The listing builds one solid part. Answer for the finished solid, in the listing's coordinates (mm). Face numbers are marked on the shaded views. A direction names the side the tool comes from. Coordinates: 2 decimals unless noted, no trailing zeros. Order: outer loops, then holes, each group sorted by start corner. A loop starts at its lowest first (then second) coordinate and runs counter-clockwise, first axis right, second up. Notation, with made-up numbers: (20.25, 42) -> (28.25, 42) arc R25 cw to (28.25, 63) -> close; hole circle Ø2 at (56, -9.5). An arc over 180 degrees is marked (long way). Return JSON: item names as keys, results as strings.
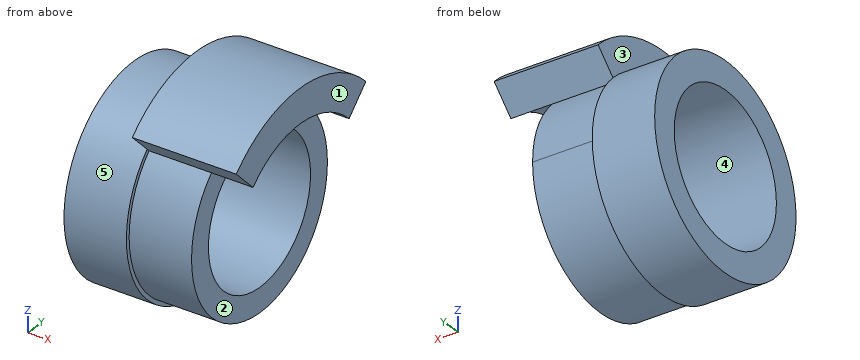
```python
from build123d import *

# Parameters (mm, degrees)
F0_R     = 38.75
F0_R_2   = 28
F1_DEPTH = 48
F5_DEPTH = 40


with BuildPart() as f1:
    # F0 (on Right) → F1 (new body)
    with BuildSketch(Plane.YZ):
        Circle(F0_R)
        Circle(F0_R_2, mode=Mode.SUBTRACT)
    extrude(amount=F1_DEPTH)

    # F2 (on Front) → F3 (revolve)
    with BuildSketch(Plane.XZ):
        Polygon((24, 50.25), (24, 38.75), (48, 38.75), (48, 37.25), (64, 37.25), (64, 50.25), align=None)
    revolve(axis=Axis((48, 0, 0), (1, 0, 0)))

    # F4 (on face) → F5 (cut)
    with BuildSketch(Plane.YZ.offset(64)):
        with BuildLine():
            ThreePointArc((37.25, 0), (-14.2549578556, -34.414512586), (-26.3397275992, 26.3397275992))
            Line((-26.3397275992, 26.3397275992), (-35.5321157546, 35.5321157546))
            ThreePointArc((-35.5321157546, 35.5321157546), (-19.2298424763, -46.4249465087), (50.25, 0))
            ThreePointArc((50.25, 0), (46.4249465087, 19.2298424763), (35.5321157546, 35.5321157546))
            Line((35.5321157546, 35.5321157546), (26.3397275992, 26.3397275992))
            ThreePointArc((26.3397275992, 26.3397275992), (34.414512586, 14.2549578556), (37.25, 0))
        make_face()
    extrude(amount=-F5_DEPTH, mode=Mode.SUBTRACT)


solid = f1.part
```
Item 1: The part is cut by section D-D on y = 22. Determine the outline of the cut face in (x, z), plus the area to 3 significant figures.
Answer list:
{"outline": "(0, -31.9) -> (24, -31.9) -> (24, -30.06) -> (48, -30.06) -> (48, -17.32) -> (0, -17.32) -> close; (0, 17.32) -> (48, 17.32) -> (48, 30.06) -> (64, 30.06) -> (64, 45.18) -> (24, 45.18) -> (24, 31.9) -> (0, 31.9) -> close", "area": "1,920 mm2"}
Item 2: Find the intervals of material crossed by probe 1 along Z at (x, y) = (22, 0); probe 2 along Z at (x, y) = (34.5, 0); probe 3 along X at (y, z) = (-4, -28), in increasing order.
Answer list:
{"probe 1": "-38.75 to -28, 28 to 38.75", "probe 2": "-37.25 to -28, 28 to 50.25", "probe 3": "0 to 48"}
Item 3: Determine the mould class of the marked faces 3, 4 and 5 for opening direction Z: pulls with the +Z half, pulls with the -Z half, needs draft (parallel to the pull), parting line crosses it, or undercut.
Answer list:
{"face 3": "needs draft", "face 4": "undercut", "face 5": "parting line crosses it"}
Item 4: Which of the six approach directions +Z, -Z, +X, -X, +Y, -Y give full straight-line access (tool end or side, diameter ignored) to the marked faces 1 and 2?
Answer list:
{"face 1": "+Z, -Z, +X, +Y, -Y", "face 2": "-Z, +X"}
Item 5: Flat-ended cylindrical pins translate along their axes: pin 1 (12 mm diameter, centred on x = 46.5, y = -15.5, fed in from -Z); pin 2 (22.5 mm diameter, centred on y = 8, z = -15.5, fed in from +X); pin 3 (12 mm diameter, centred on x = 34, z = -22.5, fed in from +Y). Find the tip coordinate at first contact, or state that the pin passes through.
Answer list:
{"pin 1": "z = -36.02", "pin 2": "x = 48", "pin 3": "y = 33.4"}
Item 6: The part is cut by section B-B on z = -5. Determine the outline of the cut face in (x, y), plus the area to 3 significant figures.
Answer list:
{"outline": "(0, -38.43) -> (24, -38.43) -> (24, -36.91) -> (48, -36.91) -> (48, -27.55) -> (0, -27.55) -> close; (0, 27.55) -> (48, 27.55) -> (48, 36.91) -> (24, 36.91) -> (24, 38.43) -> (0, 38.43) -> close", "area": "971 mm2"}
Item 7: The part is cut by section C-C on x = 25.5. Determine the outline of the cut face in (y, z).
Answer list:
{"outline": "(-35.53, 35.53) -> (-26.34, 26.34) arc R37.25 ccw (long way) to (26.34, 26.34) -> (35.53, 35.53) arc R50.25 ccw to start; hole circle Ø56 at (0, 0)"}
Item 8: The part is cut by section A-A on y = 0. Determine the outline of the cut face in (x, z), plus the area to 3 significant figures.
Answer list:
{"outline": "(0, -38.75) -> (24, -38.75) -> (24, -37.25) -> (48, -37.25) -> (48, -28) -> (0, -28) -> close; (0, 28) -> (48, 28) -> (48, 37.25) -> (64, 37.25) -> (64, 50.25) -> (24, 50.25) -> (24, 38.75) -> (0, 38.75) -> close", "area": "1,480 mm2"}
